Autodesk Inventor part; units mm, degrees
ref_plane "YZ Plane" through (0, 0, 0) normal (1, 0, 0) x (0, 1, 0)
ref_plane "XZ Plane" through (0, 0, 0) normal (0, 1, 0) x (-1, 0, 0)
ref_plane "XY Plane" through (0, 0, 0) normal (0, 0, 1) x (1, 0, 0)
sketch "Sketch1" plane through (0, 0, 0) normal (0, 0, 1) x (1, 0, 0)
  line L0 (-50.8, 66.75) -> (50.8, 66.75)
  line L1 (50.8, 66.75) -> (50.8, -66.6)
  line L2 (50.8, -66.6) -> (-50.8, -66.6)
  line L3 (-50.8, -66.6) -> (-50.8, 66.75)
  point P0 (0, 0)
  dimension "d1" = 101.6
  dimension "d2" = 133.35
  dimension "d3" = 66.75
  dimension "d4" = 50.8
extrude "Extrusion1" add sketch "Sketch1" along normal blind 100.075
sketch "Sketch2" plane through (0, 0, 100.075) normal (0, 0, 1) x (1, 0, 0)
  circle A0 centre (0, 0) radius 15.875
  dimension "d7" = 31.75
extrude "Extrusion2" add sketch "Sketch2" along normal blind 38.1
sketch "Sketch3" plane through (0, 0, 0) normal (0, 0, -1) x (-1, 0, 0)
  circle A0 centre (0, 0) radius 31.75
  dimension "d10" = 63.5
extrude "Extrusion3" add sketch "Sketch3" along normal blind 82.55
sketch "Sketch4" plane through (50.8, -66.6, 0) normal (1, 0, 0) x (0, 0, -1)
  line L0 (0, 133.35) -> (-100.075, 133.35)
  line L1 (-81.787, 133.35) -> (-18.288, 133.35)
  line L2 (-18.288, 133.35) -> (-18.288, 69.851)
  line L3 (-18.288, 69.851) -> (-81.787, 69.851)
  line L4 (-81.787, 69.851) -> (-81.787, 133.35)
  line L5 (0, 133.35) -> (0, 0)
  line L6 (-100.075, 0) -> (-100.075, 133.35)
  line L7 (0, 0) -> (-100.075, 0)
  line L8 (-81.787, 0) -> (-18.288, 0)
  line L9 (-18.288, 0) -> (-18.288, 63.499)
  line L10 (-18.288, 63.499) -> (-81.787, 63.499)
  line L11 (-81.787, 63.499) -> (-81.787, 0)
  point P0 (0, 66.6)
  dimension "d13" = 18.288
  dimension "d14" = 18.288
  dimension "d15" = 63.499
  dimension "d16" = 63.499
  dimension "d17" = 63.499
extrude "Extrusion4" add sketch "Sketch4" along normal blind 90.424 contours L2 L3 L4 L0 | L7 L11 L10 L9
sketch "Sketch5" plane through (-50.8, -66.6, 0) normal (-1, 0, 0) x (0, 0, 1)
  line L0 (18.288, 69.851) -> (18.288, 133.35)
  line L1 (18.288, 69.851) -> (81.787, 69.851)
  line L2 (18.288, 133.35) -> (81.787, 133.35)
  line L3 (81.787, 133.35) -> (81.787, 69.851)
  line L4 (81.787, 69.851) -> (18.288, 69.851)
  line L5 (18.288, 69.851) -> (18.288, 133.35)
  line L6 (18.288, 0) -> (18.288, 63.499)
  line L7 (81.787, 0) -> (81.787, 63.499)
  line L8 (18.288, 63.499) -> (81.787, 63.499)
  line L9 (81.787, 63.499) -> (81.787, 0)
  line L10 (81.787, 0) -> (18.288, 0)
  line L11 (18.288, 0) -> (18.288, 63.499)
  point P0 (0, 66.6)
extrude "Extrusion5" add sketch "Sketch5" along normal blind 90.424
sketch "Sketch7" plane through (0, 0, 138.175) normal (0, 0, 1) x (1, 0, 0)
  line L0 (-5, 13.375) -> (5, 13.375)
  line L1 (5, 13.375) -> (5, 18.375)
  line L2 (5, 18.375) -> (-5, 18.375)
  line L3 (-5, 18.375) -> (-5, 13.375)
  circle A0 centre (0, 0) radius 15.875
  line L4 (-5, 13.375) -> (5, 18.375) construction
  line L5 (5, 13.375) -> (-5, 18.375) construction
  point P0 (0, 15.875)
  point P1 (5, 15.067)
  point P2 (-5, 15.067)
  dimension "d22" = 10
  dimension "d23" = 5
extrude "Extrusion6" cut sketch "Sketch7" against normal blind 30 contours L3 A0 L1 L0 picked at (-0.5641, 14.1782)
equation "\"d16\" = d15"
equation "\"d17\" = d15"
properties part number "Semi Rotary Hydraulic Motor"
Here's how the part is built. I have some questions about the finished solid (model axes, mm). A direction names the side the tool comes from. Coordinates: 2 decimals unless noted, no trailing zeros. Order: outer loops, then holes, each group sorted by start corner. A loop starts at its lowest first (then second) coordinate and runs counter-clockwise, first axis right, second up. Notation, with made-up numbers: (51.5, 30.25) - (100.5, 30.25) arc R32 ccw to (100.5, 56.25) - close; hole circle Ø6 at (8.5, -11.75). An arc over 180 degrees is marked (long way). Use CSV: the item, a comma, the result in double quotes. Start each with the question number.
1. Suppose I cut it at A-A on x = -67. List the corners of the cut face in (y, z) for me, then the cut area to 3 significant figures.
2. Please list where these lines run through material, in increasing order: line 1 (X direction, y = 49.5, z = 1); line 2 (Y direction, x = -122, z = 19.5); line 3 (Z direction, x = -121, y = 42.5). Write a range as from..to.
3. Suppose I cut it at D-D on z = 63. List the corners of the cut face in (x, y) for me.
4. For faces 1 (the face through (-95, 35, 18.288)), 2 (the face through (95, -35, 18.288)), 3 (the face through (8.53, -13.39, 118.86)), 4 (the face through (0, 13.375, 123)), 5 (the face through (95, 3.251, 50)), which set-ups out of +Z, -Z, +X, -X, +Y, -Y let a thin tool reach every point of the face, with its end or its side?
5. Suppose I cut it at C-C on x = 0. List the corners of the cut face in (y, z) for me (3 decimals), then the cut area to 3 significant figures.
6. Suppose I cut it at B-B on y = 49.5. List the corners of the cut face in (x, z) for me (3 decimals).
7. If we mould it in two halves opening along Y, with no side actions, what happens to faces 6 (the face through (-95, 3.251, 50)), 7 (the face through (95, -3.101, 50)), 8 (the face through (95, 35, 18.288)), 9 (the face through (-2, 66.75, 49))? For each: +Y half, -Y half, draft (parallel to the pull), parting line (faces both ways), or undercut.
8. I'm going to push flat-ended pins straight in: pin 1 (2 mm diameter, centred on y = 31.5, z = 85.5, fed in from +X); pin 2 (12 mm diameter, centred on y = 29, z = 91.5, fed in from -X); pin 3 (19 mm diameter, centred on x = 88, y = 31.5, fed in from -Z); pin 4 (12 mm diameter, centred on y = -43, z = -24, fed in from -X). Where does each tip first touch, or does it pass through?
Output:
1,outline,"(-66.6, 18.29) - (-3.1, 18.29) - (-3.1, 81.79) - (-66.6, 81.79) - close; (3.25, 18.29) - (66.75, 18.29) - (66.75, 81.79) - (3.25, 81.79) - close"
1,area,"8,060 mm2"
2,line 1,"x = -50.8..50.8"
2,line 2,"y = -66.6..-3.1, 3.25..66.75"
2,line 3,"z = 18.29..81.79"
3,outline,"(-141.22, -66.6) - (141.22, -66.6) - (141.22, -3.1) - (50.8, -3.1) - (50.8, 3.25) - (141.22, 3.25) - (141.22, 66.75) - (-141.22, 66.75) - (-141.22, 3.25) - (-50.8, 3.25) - (-50.8, -3.1) - (-141.22, -3.1) - close"
4,face 1,"-Z, -X, +Y, -Y"
4,face 2,"-Z, +X, +Y, -Y"
4,face 3,"+Z"
4,face 4,"+Z, +Y"
4,face 5,"+Z, -Z, +X"
5,outline,"(-66.6, 0) - (-31.75, 0) - (-31.75, -82.55) - (31.75, -82.55) - (31.75, 0) - (66.75, 0) - (66.75, 100.075) - (15.875, 100.075) - (15.875, 108.175) - (13.375, 108.175) - (13.375, 138.175) - (-15.875, 138.175) - (-15.875, 100.075) - (-66.6, 100.075) - close"
5,area,"19,700 mm2"
6,outline,"(-141.224, 18.288) - (-50.8, 18.288) - (-50.8, 0) - (50.8, 0) - (50.8, 18.288) - (141.224, 18.288) - (141.224, 81.787) - (50.8, 81.787) - (50.8, 100.075) - (-50.8, 100.075) - (-50.8, 81.787) - (-141.224, 81.787) - close"
7,face 6,"undercut"
7,face 7,"undercut"
7,face 8,"draft"
7,face 9,"+Y half"
8,pin 1,"stops at x = 50.8"
8,pin 2,"stops at x = -50.8"
8,pin 3,"stops at z = 18.29"
8,pin 4,"passes through"
